Input: dimensioned drawing with shaded views. Units: mm. Origin: part minimum x, y, z. Round coordinates to 2 decimals unless told otherwise and drop trailing zeros. Loops run counter-clockwise (first coordinate to the right, second up) from the corner with the lowest first, then second, coordinate; pieces in that order, holes last. Notation, with made-up numbers: (-1, 13.5) -> (17, 13.5) arc R22 cw to (17, 19.5) -> close; hole circle Ø10 at (-6, 54). An arc over 180 degrees is marked (long way). Answer as a JSON object with one key per item and string values.
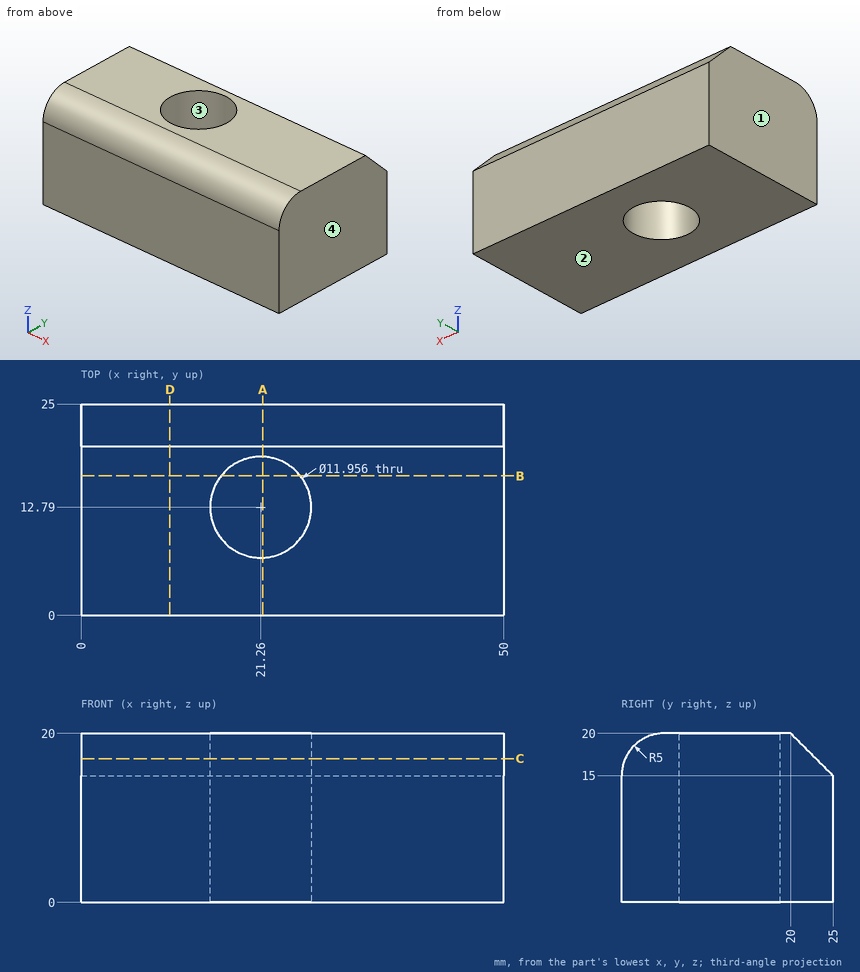
1) Section A-A, the plane x = 21.5. Output: boundary loops of the cut face in (y, z).
Output:
{"outline": "(0, 0) -> (6.82, 0) -> (6.82, 20) -> (5, 20) arc R5 ccw to (0, 15) -> close; (18.76, 0) -> (25, 0) -> (25, 15) -> (20, 20) -> (18.76, 20) -> close"}
2) Ray query, probe 1 along X at (y, z) = (12.75, 17); probe 2 along Y at (x, z) = (16, 3.5); probe 3 along X at (y, z) = (15.25, 1.25). Return the intervals inside material, ascending.
Output:
{"probe 1": "x = 0 to 15.28, 27.24 to 50", "probe 2": "y = 0 to 9.95, 15.63 to 25", "probe 3": "x = 0 to 15.81, 26.71 to 50"}
3) Section D-D, the plane x = 10.5. Output: boundary loops of the cut face in (y, z), plus the area to 3 significant figures.
Output:
{"outline": "(0, 0) -> (25, 0) -> (25, 15) -> (20, 20) -> (5, 20) arc R5 ccw to (0, 15) -> close", "area": "482 mm^2"}
4) Contact query for a flat-ended pin moving along its axis: P1, Ø9.5, axis at x = 21.26, y = 12.79, coming from the -Z side. Output: stop coordinate, or through.
Output:
{"P1": "passes through"}
5) Section C-C, the plane z = 17. Output: boundary loops of the cut face in (x, y).
Output:
{"outline": "(0, 0.42) -> (50, 0.42) -> (50, 23) -> (0, 23) -> close; hole circle Ø11.96 at (21.26, 12.79)"}
6) Section B-B, the plane y = 16.5. Output: boundary loops of the cut face in (x, z).
Output:
{"outline": "(0, 0) -> (16.57, 0) -> (16.57, 20) -> (0, 20) -> close; (25.95, 0) -> (50, 0) -> (50, 20) -> (25.95, 20) -> close"}
7) Draft query along X for the marked faces 1, 2, 3 and 4. Return one class per face: +X half, -X half, draft (parallel to the pull), parting line (faces both ways), or undercut.
Output:
{"face 1": "-X half", "face 2": "draft", "face 3": "undercut", "face 4": "+X half"}
